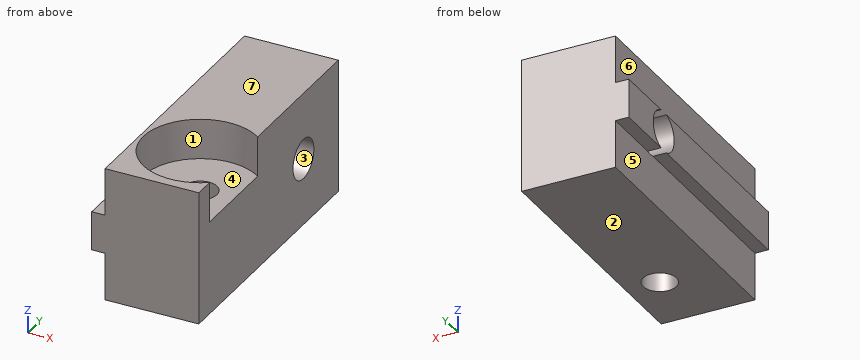
```python
from build123d import *

# Parameters (mm, degrees)
ESQUISSE1_W                      = 7
ESQUISSE1_H                      = 20
MAIN_DEPTH                       = 10
ESQUISSE4_W                      = 2.9
ESQUISSE4_H                      = 20
MAKERBEAMFIXVERTICAL_DEPTH       = 1
ESQUISSE2_R                      = 1.5
MAKERBEAMVERTICALHOLE_DEPTH      = 2
MAKERBEAMVERTICALHOLE_DEPTH_BACK = 8
SKETCH1_R                        = 1.25
CUT_EXTRUDE1_DEPTH               = 11
SKETCH2_R                        = 4.25
CUT_EXTRUDE2_DEPTH               = 3


with BuildPart() as part:
    # Esquisse1 → Main (new body)
    with BuildSketch(Plane.XY):
        with Locations((3.5, 10)):
            Rectangle(ESQUISSE1_W, ESQUISSE1_H)
    extrude(amount=MAIN_DEPTH)

    # Esquisse4 → MakerBeamFixVertical (add)
    with BuildSketch(Plane.ZY):
        with Locations((5, 10)):
            Rectangle(ESQUISSE4_W, ESQUISSE4_H)
    extrude(amount=MAKERBEAMFIXVERTICAL_DEPTH)

    # Esquisse2 → MakerBeamVerticalHole (cut, two sides)
    with BuildSketch(Plane.ZY) as makerbeamverticalhole_sk:
        with Locations((5, 15)):
            Circle(ESQUISSE2_R)
    extrude(amount=MAKERBEAMVERTICALHOLE_DEPTH, mode=Mode.SUBTRACT)
    extrude(makerbeamverticalhole_sk.sketch, amount=-MAKERBEAMVERTICALHOLE_DEPTH_BACK, mode=Mode.SUBTRACT)

    # Sketch1 → Cut-Extrude1 (cut, through all)
    with BuildSketch(Plane.XY.offset(10)):
        with Locations((4.5, 5)):
            Circle(SKETCH1_R)
    extrude(amount=-CUT_EXTRUDE1_DEPTH, mode=Mode.SUBTRACT)

    # Sketch2 → Cut-Extrude2 (cut)
    with BuildSketch(Plane.XY.offset(10)):
        with Locations((4.5, 5)):
            Circle(SKETCH2_R)
    extrude(amount=-CUT_EXTRUDE2_DEPTH, mode=Mode.SUBTRACT)


solid = part.part
```
Read the model definition and answer for the solid it produces. Units are mm, in the model's axes. Face numbers are marked on the shaded views. A direction names the side the tool comes from. Coordinates: 2 decimals unless noted, no trailing zeros. Order: outer loops, then holes, each group sorted by start corner. A loop starts at its lowest first (then second) coordinate and runs counter-clockwise, first axis right, second up. Notation, with made-up numbers: (44.5, 44.5) - (99.5, 44.5) arc R19 ccw to (99.5, 70.5) - close; hole circle Ø2 at (9.5, 54). An arc over 180 degrees is marked (long way). Answer as a JSON object with one key per item and string values. Group by question number.
Item 1: Flat-ended cylindrical pins translate along their axes: P1, Ø1.8, axis at y = 13, z = 1, coming from the -X side; P2, Ø0.5, axis at x = -0.5, y = 9.5, coming from the -Z side; P3, Ø2, axis at x = 5, y = 6.5, coming from the +Z side; P4, Ø4, axis at y = 11, z = 7.5, coming from the -X side. Find the tip coordinate at first contact, or state that the pin passes through.
Item 2: Section B-B (x = 4.5) is taken. Give the vertices of the cut face in (y, z).
Item 3: Section A-A (z = 5) is taken. Give the vertices of the cut face in (x, y), plus the area to 3 significant figures.
Item 4: Consider probe 1 along Y at (x, z) = (4.5, 5); probe 2 along Y at (x, z) = (4.5, 8.75); probe 3 along Y at (x, z) = (4.5, 4.5). Determine where each line is inside the solid, lowest interval first. Write a range as from..to.
Item 5: Section D-D (x = 2.5) is taken. Give the vertices of the cut face in (y, z).
Item 6: A tool of negligible diameter and unlimited length cuts with its end or side. For the marked faces 5, 6 and 7, from which of +Z, -Z, +X, -X, +Y, -Y can it reach the whole face along a straight path? Write none if from no direction.
Item 7: Section C-C (y = 5) is taken. Give the vertices of the cut face in (x, z).
Item 8: The mould has two halves that part along Z. Classify the marked faces 1, 2, 3 and 4: +Z half, -Z half, draft (parallel to the pull), parting line (faces both ways), or undercut.
Results are:
{
 "1": {"P1": "stops at x = 0", "P2": "stops at z = 3.55", "P3": "stops at z = 7", "P4": "stops at x = -1"},
 "2": {"outline": "(0, 0) - (3.75, 0) - (3.75, 7) - (0.75, 7) - (0.75, 10) - (0, 10) - close; (6.25, 0) - (20, 0) - (20, 10) - (9.25, 10) - (9.25, 7) - (6.25, 7) - close; hole circle Ø3 at (15, 5)"},
 "3": {"outline": "(-1, 0) - (7, 0) - (7, 13.5) - (-1, 13.5) - close; (-1, 16.5) - (7, 16.5) - (7, 20) - (-1, 20) - close; hole circle Ø2.5 at (4.5, 5)", "area": "131 mm^2"},
 "4": {"probe 1": "y = 0..3.75, 6.25..13.5, 16.5..20", "probe 2": "y = 0..0.75, 9.25..20", "probe 3": "y = 0..3.75, 6.25..13.59, 16.41..20"},
 "5": {"outline": "(0, 0) - (20, 0) - (20, 10) - (8.75, 10) - (8.75, 7) - (1.25, 7) - (1.25, 10) - (0, 10) - close; hole circle Ø3 at (15, 5)"},
 "6": {"face 5": "-Z, -X, +Y, -Y", "face 6": "+Z, -X, +Y, -Y", "face 7": "+Z, +X, -X, +Y, -Y"},
 "7": {"outline": "(-1, 3.55) - (0, 3.55) - (0, 0) - (3.25, 0) - (3.25, 7) - (0.25, 7) - (0.25, 10) - (0, 10) - (0, 6.45) - (-1, 6.45) - close; (5.75, 0) - (7, 0) - (7, 7) - (5.75, 7) - close"},
 "8": {"face 1": "draft", "face 2": "-Z half", "face 3": "undercut", "face 4": "+Z half"}
}
